The model under review builds one solid part; all positions refer to its coordinate system, in mm. Face numbers are marked on the shaded views. A direction names the side the tool comes from. Give positions to 0.01 mm unless a question says otherwise; leave off trailing zeros. Loops run counter-clockwise (first coordinate to the right, second up) from the corner with the lowest first, then second, coordinate; pieces in that order, holes last. Notation, with made-up numbers: (66, 48.25) -> (114, 48.25) arc R14 cw to (114, 67.25) -> close; hole circle Ø10 at (15, 22). An arc over 180 degrees is marked (long way). Write each question's results on one line, items separated by ' | '. Start each with the question number.
Q1. Mouldability with a two-part tool opening along Y and no side actions: class the marked faces 1, 2, 3 and 4 as released by +Y, released by -Y, zero draft, split by the parting line, or undercut.
Q2. Insertion check: pin 1 Ø5 at (x, z) = (3.5, 2) entering from +Y; pin 2 Ø0.6 at (x, z) = (0, 2) entering from +Y. Each pin has a flat end and moves straight along its axis. Give the tip position at first contact, or say it passes through.
Q3. Wall thickness on L1, parallel to Y at x = 2.75, z = 1.5; L2, parallel to X at y = 0.75, z = 3.75; L3, parallel to Y at x = -1.5, z = 2.5: over which ranges is each line inside the solid? List them lowest first. Write a range as [from, to].
Q4. We need section C-C (x = 2.5). Write out the cut boundary in (y, z), plus the area to 3 significant figures.
Q5. Machinability: for the marked faces 5, 6, 7, 8 and 9, which of the approach directions +Z, -Z, +X, -X, +Y, -Y give a long, thin tool a straight path to every point of the face, cutting with its end or side? Answer none if there is none.
Q6. We need section A-A (z = -0.5). Write out the cut boundary in (x, y).
Q7. We need section D-D (x = 4.75). Write out the cut boundary in (y, z).
Q8. We need section B-B (z = 6.25). Give the number of separate pieces and of enclosed holes in the cut face, plus the area to 3 significant figures.
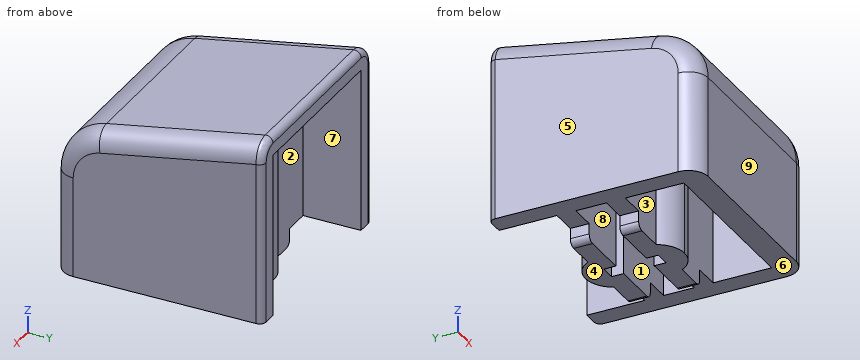
from build123d import *

# Parameters (mm, degrees)
F1_DEPTH = 14
F3_DEPTH = 16
F4_DEPTH = 16
F5_R     = 1.5
F6_DEPTH = 1.3
F7_R     = 0.5


with BuildPart() as f1:
    # F0 (on Top) → F1 (new body)
    with BuildSketch(Plane.XY):
        Polygon((6.4673761603, 1.1610865705), (6.4673761603, -1.1610865705), (4.5, -1.1610865705), (4.5, -2.5941354688), (6.4673761603, -2.5941354688), (6.4673761603, -7.0438799448), (0, -7.0438799448), (-6.4673761603, -7.0438799448), (-6.4673761603, -2.5941354688), (-4.5, -2.5941354688), (-4.5, -1.1610865705), (-6.4673761603, -1.1610865705), (-6.4673761603, 1.1610865705), (-4.5, 1.1610865705), (-4.5, 2.5941354688), (-6.4673761603, 2.5941354688), (-6.4673761603, 6.996571178), (-8, 6.996571178), (-8, -8.903428822), (8, -8.903428822), (8, 6.996571178), (6.4673761603, 6.996571178), (6.4673761603, 2.5941354688), (4.5, 2.5941354688), (4.5, 1.1610865705), align=None)
        with BuildLine():
            Line((0.5740744527, 1.1610865705), (4.5, 1.1610865705))
            Line((4.5, 1.1610865705), (4.5, 2.5941354688))
            Line((4.5, 2.5941354688), (1.9127666601, 2.5941354688))
            ThreePointArc((1.9127666601, 2.5941354688), (0, 3.7664402702), (-1.9127666601, 2.5941354688))
            Line((-1.9127666601, 2.5941354688), (-4.5, 2.5941354688))
            Line((-4.5, 2.5941354688), (-4.5, 1.1610865705))
            Line((-4.5, 1.1610865705), (-0.5740744527, 1.1610865705))
            Line((-0.5740744527, 1.1610865705), (-0.5740744527, 2.0683966577))
            Line((-0.5740744527, 2.0683966577), (0.5740744527, 2.0683966577))
            Line((0.5740744527, 2.0683966577), (0.5740744527, 1.1610865705))
        make_face()
        with BuildLine():
            Line((4.5, -2.5941354688), (4.5, -1.1610865705))
            Line((4.5, -1.1610865705), (0.5740744527, -1.1610865705))
            Line((0.5740744527, -1.1610865705), (0.5740744527, -2.0683966577))
            Line((0.5740744527, -2.0683966577), (-0.5740744527, -2.0683966577))
            Line((-0.5740744527, -2.0683966577), (-0.5740744527, -1.1610865705))
            Line((-0.5740744527, -1.1610865705), (-4.5, -1.1610865705))
            Line((-4.5, -1.1610865705), (-4.5, -2.5941354688))
            Line((-4.5, -2.5941354688), (-1.9127666601, -2.5941354688))
            ThreePointArc((-1.9127666601, -2.5941354688), (-1.1217146299, -3.4500472339), (0, -3.7664402702))
            ThreePointArc((0, -3.7664402702), (1.1217146299, -3.4500472339), (1.9127666601, -2.5941354688))
            Line((1.9127666601, -2.5941354688), (4.5, -2.5941354688))
        make_face()
    extrude(amount=F1_DEPTH)

    # F2 (on face) → F3 (intersect, through all)
    with BuildSketch(Plane(origin=(-8, 0, 0), x_dir=(0, -1, 0), z_dir=(-1, 0, 0))):
        with BuildLine():
            Line((5.36694847, 10.1407940407), (-6.996571178, 12.473533597))
            Line((-6.996571178, 12.473533597), (-6.996571178, 0))
            Line((-6.996571178, 0), (7.403428822, 0))
            Line((7.403428822, 0), (7.403428822, 7.6841399064))
            ThreePointArc((7.403428822, 7.6841399064), (6.8281104996, 9.2796336983), (5.36694847, 10.1407940407))
        make_face()
    extrude(amount=-F3_DEPTH, mode=Mode.INTERSECT)

    # F2 (on face) → F4 (join, through all)
    with BuildSketch(Plane(origin=(-8, 0, 0), x_dir=(0, -1, 0), z_dir=(-1, 0, 0))):
        with BuildLine():
            Line((5.6450602588, 11.6147865214), (-6.996571178, 14))
            Line((-6.996571178, 14), (-6.996571178, 12.473533597))
            Line((-6.996571178, 12.473533597), (5.36694847, 10.1407940407))
            ThreePointArc((5.36694847, 10.1407940407), (6.8281104996, 9.2796336983), (7.403428822, 7.6841399064))
            Line((7.403428822, 7.6841399064), (7.403428822, 0))
            Line((7.403428822, 0), (8.903428822, 0))
            Line((8.903428822, 0), (8.903428822, 7.6841399064))
            ThreePointArc((8.903428822, 7.6841399064), (7.9829195061, 10.2369299734), (5.6450602588, 11.6147865214))
        make_face()
    extrude(amount=-F4_DEPTH)

    # F5
    f5_edges = [f1.edges().sort_by_distance(p)[0] for p in [
        (-8, 0.675755, 12.807393),
        (8, 0.675755, 12.807393),
    ]]
    fillet(f5_edges, radius=F5_R)

    # F0 (on Top) → F6 (join)
    with BuildSketch(Plane.XY):
        with BuildLine():
            Line((4.5, -2.5941354688), (4.5, -1.1610865705))
            Line((4.5, -1.1610865705), (0.5740744527, -1.1610865705))
            Line((0.5740744527, -1.1610865705), (0.5740744527, -2.0683966577))
            Line((0.5740744527, -2.0683966577), (-0.5740744527, -2.0683966577))
            Line((-0.5740744527, -2.0683966577), (-0.5740744527, -1.1610865705))
            Line((-0.5740744527, -1.1610865705), (-4.5, -1.1610865705))
            Line((-4.5, -1.1610865705), (-4.5, -2.5941354688))
            Line((-4.5, -2.5941354688), (-1.9127666601, -2.5941354688))
            ThreePointArc((-1.9127666601, -2.5941354688), (-1.1217146299, -3.4500472339), (0, -3.7664402702))
            ThreePointArc((0, -3.7664402702), (1.1217146299, -3.4500472339), (1.9127666601, -2.5941354688))
            Line((1.9127666601, -2.5941354688), (4.5, -2.5941354688))
        make_face()
        with BuildLine():
            Line((0.5740744527, 1.1610865705), (4.5, 1.1610865705))
            Line((4.5, 1.1610865705), (4.5, 2.5941354688))
            Line((4.5, 2.5941354688), (1.9127666601, 2.5941354688))
            ThreePointArc((1.9127666601, 2.5941354688), (0, 3.7664402702), (-1.9127666601, 2.5941354688))
            Line((-1.9127666601, 2.5941354688), (-4.5, 2.5941354688))
            Line((-4.5, 2.5941354688), (-4.5, 1.1610865705))
            Line((-4.5, 1.1610865705), (-0.5740744527, 1.1610865705))
            Line((-0.5740744527, 1.1610865705), (-0.5740744527, 2.0683966577))
            Line((-0.5740744527, 2.0683966577), (0.5740744527, 2.0683966577))
            Line((0.5740744527, 2.0683966577), (0.5740744527, 1.1610865705))
        make_face()
    extrude(amount=-F6_DEPTH)

    # F7
    f7_edges = [f1.edges().sort_by_distance(p)[0] for p in [
        (-4.5, -1.877611, -1.3),
        (-4.5, 1.877611, -1.3),
        (4.5, -1.877611, -1.3),
        (4.5, 1.877611, -1.3),
        (0, 6.996571, 14),
    ]]
    fillet(f7_edges, radius=F7_R)


solid = f1.part
Output:
1) face 1: undercut | face 2: released by +Y | face 3: undercut | face 4: zero draft
2) pin 1: y = 3.52 | pin 2: y = 3.77
3) L1: [-8.9, -7.04], [-2.59, -1.16], [1.16, 2.59] | L2: [-8, -6.47], [6.47, 8] | L3: [-8.9, -7.04], [-3.16, -1.16], [1.16, 3.16]
4) outline: (-8.9, 0) -> (-7.04, 0) -> (-7.04, 8.98) arc R2.5 cw to (-5.37, 10.14) -> (-2.59, 10.66) -> (-2.59, -1.3) -> (-1.16, -1.3) -> (-1.16, 10.93) -> (1.16, 11.37) -> (1.16, -1.3) -> (2.59, -1.3) -> (2.59, 11.64) -> (7, 12.47) -> (7, 13.4) arc R0.5 ccw to (6.4, 13.89) -> (-5.65, 11.61) arc R4 ccw to (-8.9, 7.68) -> close | area: 76.0 mm2
5) face 5: +Z, -Z, -X, +Y, -Y | face 6: -Z, -Y | face 7: -Z, +Y | face 8: -Z | face 9: +Z, -Z, +X, -X, -Y
6) outline: (-4.5, -2.59) -> (-1.91, -2.59) arc R2.15 ccw to (1.91, -2.59) -> (4.5, -2.59) -> (4.5, -1.16) -> (0.57, -1.16) -> (0.57, -2.07) -> (-0.57, -2.07) -> (-0.57, -1.16) -> (-4.5, -1.16) -> close; (-4.5, 1.16) -> (-0.57, 1.16) -> (-0.57, 2.07) -> (0.57, 2.07) -> (0.57, 1.16) -> (4.5, 1.16) -> (4.5, 2.59) -> (1.91, 2.59) arc R2.15 ccw to (-1.91, 2.59) -> (-4.5, 2.59) -> close
7) outline: (-8.9, 0) -> (-7.04, 0) -> (-7.04, 8.98) arc R2.5 cw to (-5.37, 10.14) -> (-2.59, 10.66) -> (-2.59, 0) -> (-1.16, 0) -> (-1.16, 10.93) -> (1.16, 11.37) -> (1.16, 0) -> (2.59, 0) -> (2.59, 11.64) -> (7, 12.47) -> (7, 13.4) arc R0.5 ccw to (6.4, 13.89) -> (-5.65, 11.61) arc R4 ccw to (-8.9, 7.68) -> close
8) separate pieces: 1 | enclosed holes: 2 | area: 113 mm2
